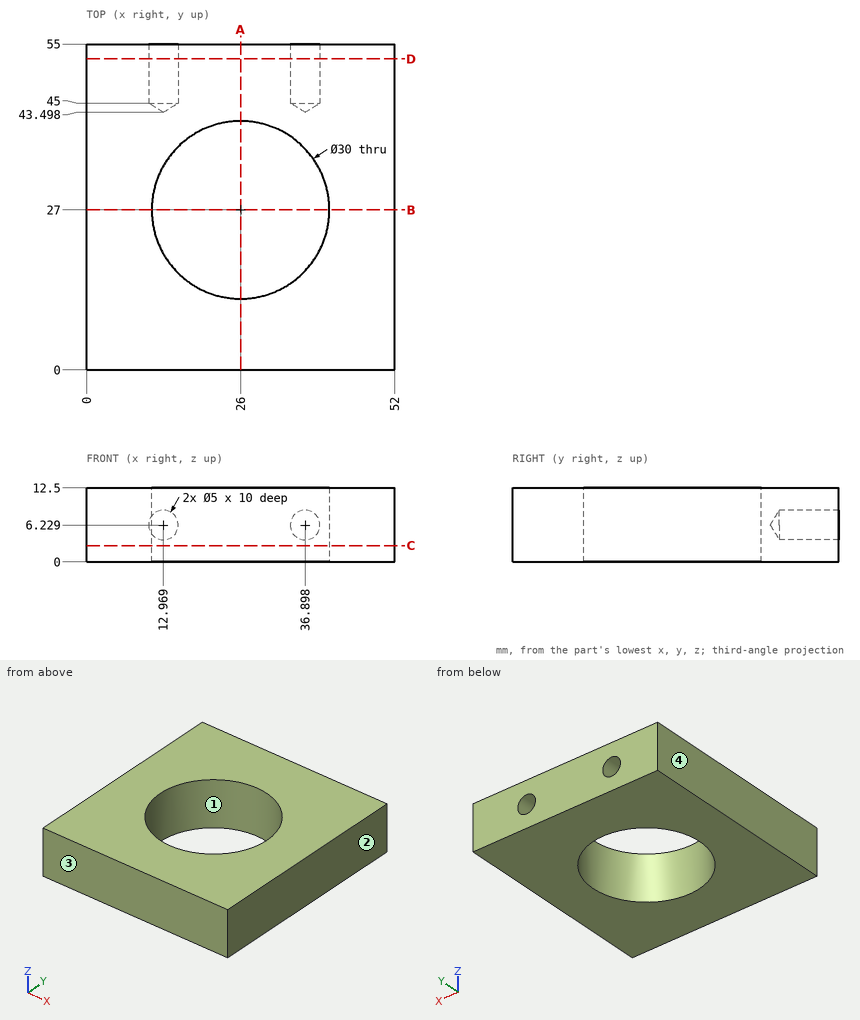
Job drawing, mm, ordinate dimensions from the low corner. One solid piece. Give positions to 0.01 mm unless a question says otherwise; leave off trailing zeros. Order: outer loops, then holes, each group sorted by start corner. A loop starts at its lowest first (then second) coordinate and runs counter-clockwise, first axis right, second up. Notation, with made-up numbers: (26, 6) - (34, 6) arc R19 cw to (34, 23) - close; hole circle Ø10 at (10.25, -10.5). An arc over 180 degrees is marked (long way). Answer in a Markdown table with one row per item.
1. Pull direction X, two halves, no side cores. Call the marked faces 1, 2, 3 and 4: pulls with the +X half, pulls with the -X half, needs draft (parallel to the pull), parting line crosses it, or undercut.
Data:
| item | result |
|---|---|
| face 1 | undercut |
| face 2 | pulls with the +X half |
| face 3 | needs draft |
| face 4 | pulls with the -X half |
2. Probe probe 1 along Y at (x, z) = (26, 8.75); probe 2 along X at (y, z) = (46.5, 7.25) (1 decimal); probe 3 along X at (y, z) = (35.5, 6). List the from-to ranges inside material, lowest first. Write a range as [from, to].
Data:
| item | result |
|---|---|
| probe 1 | y = [0, 12], [42, 55] |
| probe 2 | x = [0, 10.7], [15.3, 34.6], [39.2, 52] |
| probe 3 | x = [0, 13.64], [38.36, 52] |
3. Saw through at B-B, the plane y = 27. Give the cut face in (x, z).
Data:
| item | result |
|---|---|
| outline | (0, 0) - (11, 0) - (11, 12.5) - (0, 12.5) - close; (41, 0) - (52, 0) - (52, 12.5) - (41, 12.5) - close |
4. Saw through at D-D, the plane y = 52.5. Give the cut face in (x, z).
Data:
| item | result |
|---|---|
| outline | (0, 0) - (52, 0) - (52, 12.5) - (0, 12.5) - close; hole circle Ø5 at (12.97, 6.23); hole circle Ø5 at (36.9, 6.23) |
5. Saw through at C-C, the plane z = 2.75. Give the cut face in (x, y).
Data:
| item | result |
|---|---|
| outline | (0, 0) - (52, 0) - (52, 55) - (0, 55) - close; hole circle Ø30 at (26, 27) |
6. Saw through at A-A, the plane x = 26. Give the cut face in (y, z).
Data:
| item | result |
|---|---|
| outline | (0, 0) - (12, 0) - (12, 12.5) - (0, 12.5) - close; (42, 0) - (55, 0) - (55, 12.5) - (42, 12.5) - close |
